from build123d import *

# Parameters (mm, degrees)
BOSS_EXTRU_1_DEPTH           = 1.5
ESQUISSE2_W                  = 40
ESQUISSE2_H                  = 40
BOSS_EXTRU_2_DEPTH           = 1.5
ENL_V_MAT_EXTRU_1_DEPTH      = 111.344913793
ENL_V_MAT_EXTRU_1_DEPTH_BACK = 111.344913793
ESQUISSE3_W                  = 1.5
ESQUISSE3_H                  = 60
ENL_V_MAT_EXTRU_2_DEPTH      = 111.344913793
ENL_V_MAT_EXTRU_2_DEPTH_BACK = 111.344913793
ESQUISSE4_R                  = 1.75
ESQUISSE4_R_2                = 2
ENL_V_MAT_EXTRU_3_DEPTH      = 111.582548352
ENL_V_MAT_EXTRU_3_DEPTH_BACK = 111.582548352
ESQUISSE5_R                  = 3.5
ESQUISSE14_W                 = 3
ESQUISSE14_H                 = 2
ENL_V_MAT_EXTRU_4_DEPTH      = 111.344913793
CONG_4_R                     = 1
CONG_5_R                     = 3
CONVERTIR_VOLUME2_DEPTH      = 40
CONVERTIR_VOLUME2_2_DEPTH    = 40


# Read off the part's stored shape, not the designer's step: Convertir-Volume2
with BuildPart() as part:
    # Esquisse1 → Boss.-Extru.1 (new body)
    with BuildSketch(Plane.XY):
        Polygon((0, 0), (0, 100), (24, 100), (24, 14), (10, 0), align=None)
    extrude(amount=BOSS_EXTRU_1_DEPTH)

    # Esquisse2 → Boss.-Extru.2 (add)
    with BuildSketch(Plane.ZY):
        with Locations((21.5, 20)):
            Rectangle(ESQUISSE2_W, ESQUISSE2_H)
    extrude(amount=-BOSS_EXTRU_2_DEPTH)

    # Esquisse3 → Enlèv. mat.-Extru.1 (cut, two sides: drawn at the far end of the back side and taken through both)
    with BuildSketch(Plane.XY.offset(1.5).offset(-ENL_V_MAT_EXTRU_1_DEPTH_BACK)):
        with Locations((0.75, 70)):
            Rectangle(ESQUISSE3_W, ESQUISSE3_H)
    extrude(amount=ENL_V_MAT_EXTRU_1_DEPTH + ENL_V_MAT_EXTRU_1_DEPTH_BACK, mode=Mode.SUBTRACT)

    # Esquisse4 → Enlèv. mat.-Extru.2 (cut, two sides: drawn at the far end of the back side and taken through both)
    with BuildSketch(Plane.XY.offset(1.5).offset(-ENL_V_MAT_EXTRU_2_DEPTH_BACK)):
        with Locations((5.25, 67.5)):
            Circle(ESQUISSE4_R)
        with Locations(Location((20.25, 67.5, 0), (0, 0, 180))):
            Circle(ESQUISSE4_R)
        with Locations((7.75, 27.5)):
            Circle(ESQUISSE4_R_2)
        with Locations(Location((17.75, 27.5, 0), (0, 0, 180))):
            Circle(ESQUISSE4_R_2)
    extrude(amount=ENL_V_MAT_EXTRU_2_DEPTH + ENL_V_MAT_EXTRU_2_DEPTH_BACK, mode=Mode.SUBTRACT)

    # Esquisse5 → Enlèv. mat.-Extru.3 (cut, two sides: drawn at the far end of the back side and taken through both)
    with BuildSketch(Plane(origin=(1.5, 0, 0), x_dir=(0, 0, -1), z_dir=(1, 0, 0)).offset(-ENL_V_MAT_EXTRU_3_DEPTH_BACK)):
        with Locations((-34, 20)):
            Circle(ESQUISSE5_R)
        with Locations((-9, 20)):
            Circle(ESQUISSE5_R)
    extrude(amount=ENL_V_MAT_EXTRU_3_DEPTH + ENL_V_MAT_EXTRU_3_DEPTH_BACK, mode=Mode.SUBTRACT)

    # Esquisse14 → Enlèv. mat.-Extru.4 (cut, through all)
    with BuildSketch(Plane.XY.offset(1.5)):
        with Locations((3, 41)):
            Rectangle(ESQUISSE14_W, ESQUISSE14_H)
    extrude(amount=-ENL_V_MAT_EXTRU_4_DEPTH, mode=Mode.SUBTRACT)

    # Congé4
    cong_4_edges = [part.edges().sort_by_distance(p)[0] for p in [
        (1.5, 42, 0.75),
        (4.5, 42, 0.75),
        (4.5, 40, 0.75),
    ]]
    fillet(cong_4_edges, radius=CONG_4_R - 0.0001)  # a hair under: the kernel refuses the full size

    # Congé5
    cong_5_edges = [part.edges().sort_by_distance(p)[0] for p in [
        (0.75, 40, 41.5),
        (0.75, 0, 41.5),
        (1.5, 100, 0.75),
        (24, 100, 0.75),
        (24, 14, 0.75),
        (10, 0, 0.75),
    ]]
    fillet(cong_5_edges, radius=CONG_5_R)

    # Convertir-Volume2 outline → Convertir-Volume2 (cut)
    with BuildSketch(Plane(origin=(0, 0, 0), x_dir=(1, 0, 0), z_dir=(0, 1, 0))):
        with BuildLine():
            Line((0, 0), (0, -3))
            ThreePointArc((0, -3), (0.878679656, -0.878679656), (3, 0))
            Line((3, 0), (0, 0))
        make_face()
    extrude(amount=CONVERTIR_VOLUME2_DEPTH, mode=Mode.SUBTRACT)

    # Convertir-Volume2 2 outline → Convertir-Volume2 2 (add)
    with BuildSketch(Plane(origin=(0, 0, 0), x_dir=(1, 0, 0), z_dir=(0, 1, 0))):
        with BuildLine():
            Line((1.5, -1.5), (1.5, -3))
            ThreePointArc((1.5, -3), (1.939339828, -1.939339828), (3, -1.5))
            Line((3, -1.5), (1.5, -1.5))
        make_face()
    extrude(amount=CONVERTIR_VOLUME2_2_DEPTH)


solid = part.part
Check sheet for the modelled part. Datum: model origin and axes. Units: mm. A direction names the side the tool comes from. Round coordinates to 2 decimals unless told otherwise and drop trailing zeros. Write each loop counter-clockwise with the first axis right and the second up, starting at its lowest first coordinate (ties: lowest second). Pieces come first, ordered by that corner, then holes. Notation, with made-up numbers: (64.5, 38.25) - (101.5, 38.25) arc R13 ccw to (101.5, 58.25) - close; hole circle Ø9 at (46.25, -39). An arc over 180 degrees is marked (long way). Return JSON: item names as keys, results as strings.
Q1. Cross-section at C-C (x = 13.75). Record the boundary of the cut face in (y, z), then the cut area to 3 significant figures.
Returned:
{"outline": "(3.75, 0) - (100, 0) - (100, 1.5) - (3.75, 1.5) - close", "area": "144 mm²"}
Q2. Scan lines: L1, parallel to Y at x = 0.7, z = 9; L2, parallel to Z at x = 0.55, y = 20; L3, parallel to Y at x = 7.75, z = 0.45. Record each from-to range of solid material in increasing order. Write a range as from..to.
Returned:
{"L1": "y = 0..16.5, 23.5..40", "L2": "z = 1.27..5.5, 12.5..30.5, 37.5..41.5", "L3": "y = 0..25.5, 29.5..100"}
Q3. Cross-section at D-D (y = 67.5). Record the boundary of the cut face in (x, z), then the cut area to 4 significant figures.
Returned:
{"outline": "(1.5, 0) - (3.5, 0) - (3.5, 1.5) - (1.5, 1.5) - close; (7, 0) - (18.5, 0) - (18.5, 1.5) - (7, 1.5) - close; (22, 0) - (24, 0) - (24, 1.5) - (22, 1.5) - close", "area": "23.25 mm²"}
Q4. Draft check along X on faces 4 (the flat face through (17, 7, 1)), 5 (the cylindrical face through (7.316, 25.548, 0.74)), 6 (the flat face through (0, 20, 22)), 7 (the cylindrical face through (0.76, 39.14, 40.6)). Enter one of: released by +X, released by -X, zero draft, split by the parting line, or undercut.
Returned:
{"face 4": "released by +X", "face 5": "undercut", "face 6": "released by -X", "face 7": "zero draft"}
Q5. Cross-section at A-A (y = 27.5). Record the boundary of the cut face in (x, z).
Returned:
{"outline": "(0, 3) arc R3 ccw to (3, 0) - (5.75, 0) - (5.75, 1.5) - (3, 1.5) arc R1.5 cw to (1.5, 3) - (1.5, 41.5) - (0, 41.5) - close; (9.75, 0) - (15.75, 0) - (15.75, 1.5) - (9.75, 1.5) - close; (19.75, 0) - (24, 0) - (24, 1.5) - (19.75, 1.5) - close"}
Q6. Depth check by flat-ended pin: P1, Ø8, axis at x = 9, y = 80.5, coming from the +Z side; P2, Ø1.8, axis at x = 1, z = 21, coming from the +Y side; P3, Ø4, axis at y = 10.5, z = 8.5, coming from the +X side. Enter the tip coordinate at first touch or a pass-through.
Returned:
{"P1": "stops at z = 1.5", "P2": "stops at y = 40", "P3": "stops at x = 1.5"}
Q7. Cross-section at B-B (z = 9). Record the boundary of the cut face in (x, y), then the cut area to 3 significant figures.
Returned:
{"outline": "(0, 0) - (1.5, 0) - (1.5, 16.5) - (0, 16.5) - close; (0, 23.5) - (1.5, 23.5) - (1.5, 40) - (0, 40) - close", "area": "49.5 mm²"}
Q8. Access from +Z, -Z, +X, -X, +Y, -Y to the whole of each face (thin tool, end or side, straight path). Record for faces 1 (the cylindrical face through (23.14, 99.1, 0.76)), 2 (the flat face through (1.5, 20, 22)), 3 (the cylindrical face through (0.86, 19.72, 0.9)).
Returned:
{"face 1": "+Z, -Z, +X, +Y", "face 2": "+Z, +X, +Y, -Y", "face 3": "-Z, -X, -Y"}
